Answer from the drawing. Dimensions are ordinates in mm from the lowest x, y and z of the part. Coordinates: 2 decimals unless noted, no trailing zeros. Write each loop counter-clockwise with the first axis right and the second up, starting at its lowest first coordinate (ties: lowest second). Pieces come first, ordered by that corner, then holes. Notation, with made-up numbers: (59, -37.5) -> (63, -37.5) arc R14 cw to (63, -18.5) -> close; hole circle Ø9 at (25.25, 70.25). An arc over 180 degrees is marked (long way). Return JSON: item names as keys, results as strings.
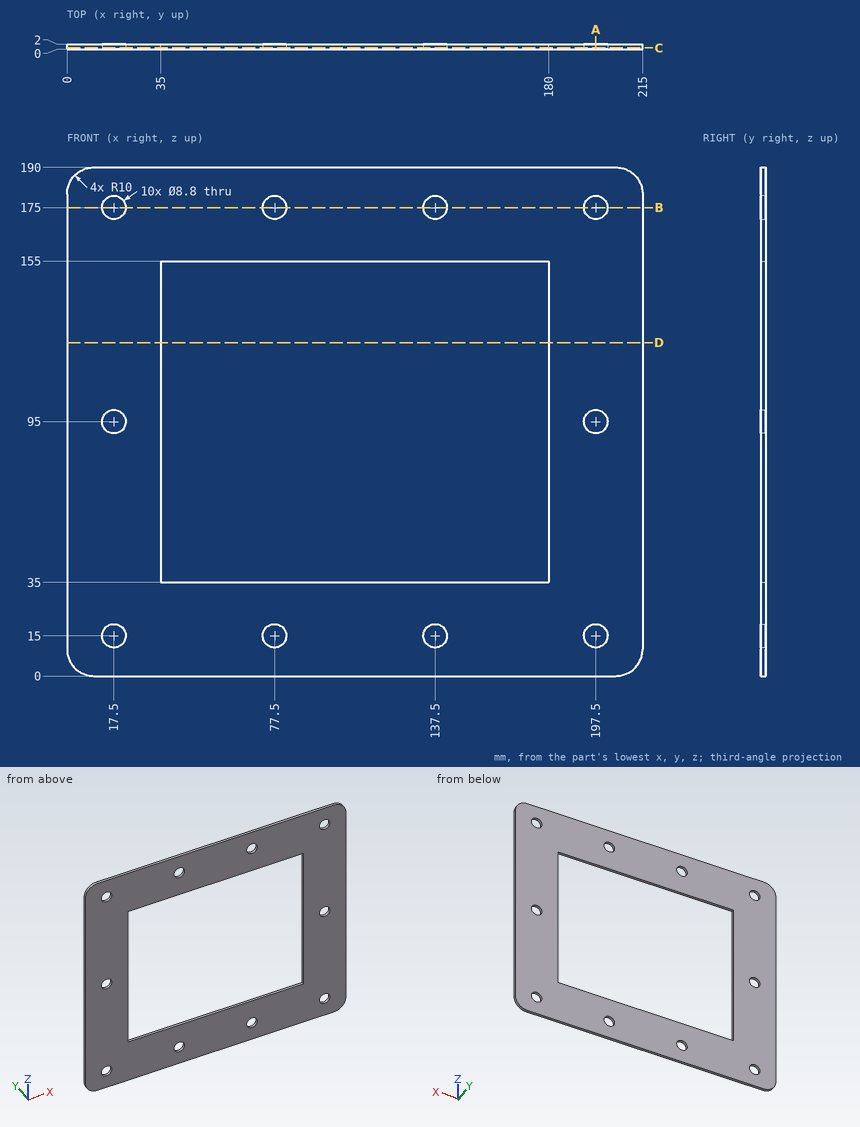
1. A flat-ended cylindrical pin translates along its axis: pin 1 Ø10 at (x, z) = (137.5, 175) entering from +Y. Find the tip coordinate at first contact, or state that the pin passes through.
Taken from the geometry:
{"pin 1": "stops at y = 2"}
2. The part is cut by section D-D (z = 124.5). Determine the outline of the cut face in (x, y).
Taken from the geometry:
{"outline": "(0, 0) -> (35, 0) -> (35, 2) -> (0, 2) -> close; (180, 0) -> (215, 0) -> (215, 2) -> (180, 2) -> close"}
3. The part is cut by section C-C (y = 0.55). Count the separate pieces of the cut face and the enclosed holes in it, then the cut area to 3 significant figures.
Taken from the geometry:
{"separate pieces": "1", "enclosed holes": "11", "area": "22,800 mm2"}
4. The part is cut by section B-B (z = 175). Determine the outline of the cut face in (x, y).
Taken from the geometry:
{"outline": "(0, 0) -> (13.1, 0) -> (13.1, 2) -> (0, 2) -> close; (21.9, 0) -> (73.1, 0) -> (73.1, 2) -> (21.9, 2) -> close; (81.9, 0) -> (133.1, 0) -> (133.1, 2) -> (81.9, 2) -> close; (141.9, 0) -> (193.1, 0) -> (193.1, 2) -> (141.9, 2) -> close; (201.9, 0) -> (215, 0) -> (215, 2) -> (201.9, 2) -> close"}
5. Consider L1, parallel to X at y = 1.3, z = 175; L2, parallel to X at y = 0.8, z = 95; L3, parallel to Z at x = 197.5, y = 1.45. Determine where each line is inside the solid, lowest interval first.
Taken from the geometry:
{"L1": "x = 0 to 13.1, 21.9 to 73.1, 81.9 to 133.1, 141.9 to 193.1, 201.9 to 215", "L2": "x = 0 to 13.1, 21.9 to 35, 180 to 193.1, 201.9 to 215", "L3": "z = 0 to 10.6, 19.4 to 90.6, 99.4 to 170.6, 179.4 to 190"}
6. The part is cut by section A-A (x = 197.5). Determine the outline of the cut face in (y, z).
Taken from the geometry:
{"outline": "(0, 0) -> (2, 0) -> (2, 10.6) -> (0, 10.6) -> close; (0, 19.4) -> (2, 19.4) -> (2, 90.6) -> (0, 90.6) -> close; (0, 99.4) -> (2, 99.4) -> (2, 170.6) -> (0, 170.6) -> close; (0, 179.4) -> (2, 179.4) -> (2, 190) -> (0, 190) -> close"}
